Verification items for the finished model (mm, model axes). A direction names the side the tool comes from. Give positions to 0.01 mm unless a question says otherwise; leave off trailing zeros.
from build123d import *

# Parameters (mm, degrees)
SKETCH1_R                                  = 87.5
BOSS_EXTRUDE1_DEPTH                        = 2
SKETCH3_R                                  = 1.75
CUT_EXTRUDE1_DEPTH                         = 124.759848093
MIRROR1_AT_THE_SECOND_PLANE_COPY_1_SKETC_R = 1.75
MIRROR1_AT_THE_SECOND_PLANE_COPY_1_DEPTH   = 124.759848093
CUT_EXTRUDE2_DEPTH                         = 124.759848093
CUT_EXTRUDE2_DEPTH_BACK                    = 124.759848093
SKETCH4_W                                  = 55
SKETCH4_H                                  = 40
SKETCH5_R                                  = 1.75
CUT_EXTRUDE3_DEPTH                         = 124.759848093
SKETCH8_W                                  = 50
SKETCH8_H                                  = 15
CUT_EXTRUDE4_DEPTH                         = 124.759848093
SKETCH9_R                                  = 1.75
CUT_EXTRUDE5_DEPTH                         = 124.759848093
CIRPATTERN1_COUNT                          = 3
CIRPATTERN1_ANGLE                          = 180
SKETCH10_W                                 = 30
SKETCH10_H                                 = 10
CUT_EXTRUDE6_DEPTH                         = 124.759848093
SKETCH11_R                                 = 1.75
CUT_EXTRUDE7_DEPTH                         = 124.759848093
SKETCH12_R                                 = 1.75
CUT_EXTRUDE8_DEPTH                         = 124.759848093
SKETCH13_R                                 = 1.75
CUT_EXTRUDE9_DEPTH                         = 124.759848093


with BuildPart() as part:
    # Sketch1 → Boss-Extrude1 (new body)
    with BuildSketch(Plane.XY):
        Circle(SKETCH1_R)
    extrude(amount=-BOSS_EXTRUDE1_DEPTH)

    # Sketch3 → Cut-Extrude1 (cut, through all)
    with BuildSketch(Plane.XY):
        with BuildLine():
            Line((-62.036781461, 31.168523814), (-49.014025927, 20.241134449))
            Line((-49.014025927, 20.241134449), (-28.444822418, 44.754556629))
            Line((-28.444822418, 44.754556629), (-41.467577951, 55.681945993))
            Line((-41.467577951, 55.681945993), (-37.289458488, 60.661234874))
            Line((-37.289458488, 60.661234874), (-50.312214021, 71.588624238))
            ThreePointArc((-50.312214021, 71.588624238), (-67.028888773, 56.243915848), (-79.237656457, 37.116624298))
            Line((-79.237656457, 37.116624298), (-66.214900923, 26.189234933))
            Line((-66.214900923, 26.189234933), (-62.036781461, 31.168523814))
        make_face()
        with Locations((-61.645137707, 14.522304568)):
            Circle(SKETCH3_R)
        with Locations((-25.006243955, 58.186837826)):
            Circle(SKETCH3_R)
    cut_extrude1 = extrude(amount=-CUT_EXTRUDE1_DEPTH, mode=Mode.SUBTRACT)

    # Mirror1: Cut-Extrude1 across plane
    add(cut_extrude1.mirror(Plane(origin=(0, 0, 0), x_dir=(0, 0, 1), z_dir=(1, 0, 0))), mode=Mode.SUBTRACT)

    # Mirror1 at the second plane: Cut-Extrude1 across plane
    add(cut_extrude1.mirror(Plane.ZX), mode=Mode.SUBTRACT)

    # Mirror1 at the second plane copy 1 sketc → Mirror1 at the second plane copy 1 (cut, through all)
    with BuildSketch(Plane(origin=(0, 0, 0), x_dir=(-1, 0, 0), z_dir=(0, 0, 1))):
        with BuildLine():
            Line((-62.036781461, 31.168523814), (-49.014025927, 20.241134449))
            Line((-49.014025927, 20.241134449), (-28.444822418, 44.754556629))
            Line((-28.444822418, 44.754556629), (-41.467577951, 55.681945993))
            Line((-41.467577951, 55.681945993), (-37.289458488, 60.661234874))
            Line((-37.289458488, 60.661234874), (-50.312214021, 71.588624238))
            ThreePointArc((-50.312214021, 71.588624238), (-67.028888773, 56.243915848), (-79.237656457, 37.116624298))
            Line((-79.237656457, 37.116624298), (-66.214900923, 26.189234933))
            Line((-66.214900923, 26.189234933), (-62.036781461, 31.168523814))
        make_face()
        with Locations((-61.645137707, 14.522304568)):
            Circle(MIRROR1_AT_THE_SECOND_PLANE_COPY_1_SKETC_R)
        with Locations((-25.006243955, 58.186837826)):
            Circle(MIRROR1_AT_THE_SECOND_PLANE_COPY_1_SKETC_R)
    extrude(amount=-MIRROR1_AT_THE_SECOND_PLANE_COPY_1_DEPTH, mode=Mode.SUBTRACT)

    # Sketch4 → Cut-Extrude2 (cut, two sides: drawn at the far end of the back side and taken through both)
    with BuildSketch(Plane.XY.offset(-CUT_EXTRUDE2_DEPTH_BACK)):
        with Locations((0, 87.5)):
            Rectangle(SKETCH4_W, SKETCH4_H)
    extrude(amount=CUT_EXTRUDE2_DEPTH + CUT_EXTRUDE2_DEPTH_BACK, mode=Mode.SUBTRACT)

    # Sketch5 → Cut-Extrude3 (cut, through all)
    with BuildSketch(Plane.XY):
        with Locations((-50, 15)):
            Circle(SKETCH5_R)
        with Locations((-50, -15)):
            Circle(SKETCH5_R)
    cut_extrude3 = extrude(amount=-CUT_EXTRUDE3_DEPTH, mode=Mode.SUBTRACT)

    # Sketch8 → Cut-Extrude4 (cut, through all)
    with BuildSketch(Plane.XY):
        with Locations((-55, 0)):
            Rectangle(SKETCH8_W, SKETCH8_H)
    cut_extrude4 = extrude(amount=-CUT_EXTRUDE4_DEPTH, mode=Mode.SUBTRACT)

    # Sketch9 → Cut-Extrude5 (cut, through all)
    with BuildSketch(Plane.XY):
        with Locations((-35, 10.5)):
            Circle(SKETCH9_R)
        with Locations((-35, -10.5)):
            Circle(SKETCH9_R)
        with Locations((-55, 10.5)):
            Circle(SKETCH9_R)
        with Locations((-55, -10.5)):
            Circle(SKETCH9_R)
        with Locations((-75, 10.5)):
            Circle(SKETCH9_R)
        with Locations((-75, -10.5)):
            Circle(SKETCH9_R)
    cut_extrude5 = extrude(amount=-CUT_EXTRUDE5_DEPTH, mode=Mode.SUBTRACT)

    # CirPattern1: Cut-Extrude3, Cut-Extrude4, Cut-Extrude5 ×3 about axis
    cirpattern1_axis = Axis((0, 0, 0), (0, 0, 1))
    add([cut_extrude3.rotate(cirpattern1_axis, i * CIRPATTERN1_ANGLE / (CIRPATTERN1_COUNT - 1)) for i in range(1, CIRPATTERN1_COUNT)], mode=Mode.SUBTRACT)
    add([cut_extrude4.rotate(cirpattern1_axis, i * CIRPATTERN1_ANGLE / (CIRPATTERN1_COUNT - 1)) for i in range(1, CIRPATTERN1_COUNT)], mode=Mode.SUBTRACT)
    add([cut_extrude5.rotate(cirpattern1_axis, i * CIRPATTERN1_ANGLE / (CIRPATTERN1_COUNT - 1)) for i in range(1, CIRPATTERN1_COUNT)], mode=Mode.SUBTRACT)

    # Sketch10 → Cut-Extrude6 (cut, through all)
    with BuildSketch(Plane.XY):
        with Locations((0, 52.5)):
            Rectangle(SKETCH10_W, SKETCH10_H)
    extrude(amount=-CUT_EXTRUDE6_DEPTH, mode=Mode.SUBTRACT)

    # Sketch11 → Cut-Extrude7 (cut, through all)
    with BuildSketch(Plane.XY):
        with Locations((-15, 42.5)):
            Circle(SKETCH11_R)
        with Locations((15, 42.5)):
            Circle(SKETCH11_R)
        with Locations((-15, 36.5)):
            Circle(SKETCH11_R)
        with Locations((15, 36.5)):
            Circle(SKETCH11_R)
        with Locations((-15, 30.5)):
            Circle(SKETCH11_R)
        with Locations((15, 30.5)):
            Circle(SKETCH11_R)
        with Locations((-15, 24.5)):
            Circle(SKETCH11_R)
        with Locations((15, 24.5)):
            Circle(SKETCH11_R)
        with Locations((-15, 18.5)):
            Circle(SKETCH11_R)
        with Locations((15, 18.5)):
            Circle(SKETCH11_R)
        with Locations((-15, 12.5)):
            Circle(SKETCH11_R)
        with Locations((15, 12.5)):
            Circle(SKETCH11_R)
        with Locations((-15, 6.5)):
            Circle(SKETCH11_R)
        with Locations((15, 6.5)):
            Circle(SKETCH11_R)
        with Locations((-15, 0.5)):
            Circle(SKETCH11_R)
        with Locations((15, 0.5)):
            Circle(SKETCH11_R)
    extrude(amount=-CUT_EXTRUDE7_DEPTH, mode=Mode.SUBTRACT)

    # Sketch12 → Cut-Extrude8 (cut, through all)
    with BuildSketch(Plane.XY):
        with Locations((-77.524641215, 28.216661824)):
            Circle(SKETCH12_R)
        with Locations((-81.246639624, 14.325974658)):
            Circle(SKETCH12_R)
        with Locations((-82.5, 0)):
            Circle(SKETCH12_R)
        with Locations((-81.246639624, -14.325974658)):
            Circle(SKETCH12_R)
        with Locations((-77.524641215, -28.216661824)):
            Circle(SKETCH12_R)
    cut_extrude8 = extrude(amount=-CUT_EXTRUDE8_DEPTH, mode=Mode.SUBTRACT)

    # Mirror2: Cut-Extrude8 across plane
    add(cut_extrude8.mirror(Plane(origin=(0, 0, 0), x_dir=(0, 0, 1), z_dir=(1, 0, 0))), mode=Mode.SUBTRACT)

    # Sketch13 → Cut-Extrude9 (cut, through all)
    with BuildSketch(Plane.XY):
        with Locations((-41.25, -71.447095812)):
            Circle(SKETCH13_R)
        with Locations((-28.216661824, -77.524641215)):
            Circle(SKETCH13_R)
        with Locations((-14.325974658, -81.246639624)):
            Circle(SKETCH13_R)
        with Locations((0, -82.5)):
            Circle(SKETCH13_R)
        with Locations((14.325974658, -81.246639624)):
            Circle(SKETCH13_R)
        with Locations((28.216661824, -77.524641215)):
            Circle(SKETCH13_R)
        with Locations((41.25, -71.447095812)):
            Circle(SKETCH13_R)
    extrude(amount=-CUT_EXTRUDE9_DEPTH, mode=Mode.SUBTRACT)


solid = part.part
(1) Set-up check for faces 1 (the flat face through (39.408, -58.137, -0.986)), 2 (the flat face through (38.87, -32.33, -0.99)), 3 (the flat face through (72.82, 31.73, -0.99)), 4 (the flat face through (-43.71, 66.05, -0.99)), 5 (the flat face through (-72.82, -31.73, -0.99)): record each of +Z, -Z, +X, -X, +Y, -Y from which the full face is reachable in a straight line by a thin tool's end or side.
Solved:
face 1: +Z, -Z, +X
face 2: +Z, -Z
face 3: +Z, -Z, +Y
face 4: +Z, -Z, -X
face 5: +Z, -Z, -Y
(2) Release check for a two-part mould opening along Y. For faces 6 (the flat face through (34.865, -50.142, -0.986)), 7 (the flat face through (64.16, 28.64, -0.99)), 8 (the flat face through (-1, -1, -2)) record: pulls with the +Y half, pulls with the -Y half, needs draft (parallel to the pull), parting line crosses it, or undercut.
Solved:
face 6: undercut
face 7: pulls with the +Y half
face 8: needs draft
(3) Scan lines: line 1 (X direction, y = -2.5, z = -0.45); line 2 (Y direction, x = 32.5, z = -1.3); line 3 (Y direction, x = -36, z = -0.6). Record each from-to range of solid material in increasing order.
Solved:
line 1: x = -87.46 to -80, -30 to 30, 80 to 87.46
line 2: y = -81.24 to -48.16, -39.92 to -7.5, 7.5 to 39.92, 48.16 to 81.24
line 3: y = -79.75 to -51.09, -35.75 to -11.94, -9.06 to -7.5, 7.5 to 9.06, 11.94 to 35.75, 51.09 to 79.75
(4) Go/stop test with flat-tipped pins: pin 1 (4.5 mm diameter, centred on x = -10.5, y = -55, fed in from -Z); pin 2 (3 mm diameter, centred on x = 10.5, y = -75, fed in from +Z); pin 3 (1 mm diameter, centred on x = -44, z = -1.5, fed in from +Y). Record where each tip stops, or that it passes through.
Solved:
pin 1: stops at z = -2
pin 2: passes through
pin 3: stops at y = 75.92
(5) Section check A-A, the plane z = -0.45. Give the number of separate pieces and of enclosed holes in the cut face, then the cut area to 3 significant figures.
Solved:
separate pieces: 1
enclosed holes: 69
area: 14,300 mm2
